Design review of the part shown in the three views and the two pictorial views. Dimensions are in mm from the part's minimum x, y and z. A direction names the side the tool comes from. Give positions to 0.01 mm unless a question says otherwise; leave off trailing zeros. Order: outer loops, then holes, each group sorted by start corner. A loop starts at its lowest first (then second) coordinate and runs counter-clockwise, first axis right, second up. Notation, with made-up numbers: (75.5, 37) - (107.5, 37) arc R30 ccw to (107.5, 64) - close; hole circle Ø10 at (18.5, -25.5). An arc over 180 degrees is marked (long way). Put each result on its own line as item: value.
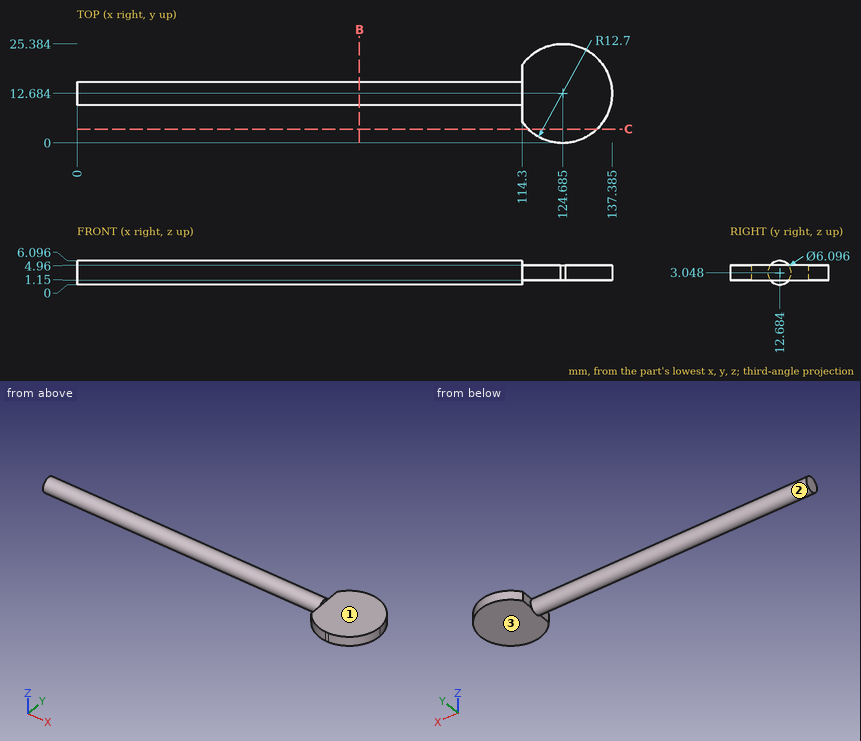
(1) Take a section at C-C, the plane y = 3.5. Write out the cut boundary in (x, z).
The answers:
outline: (115.91, 1.15) - (133.46, 1.15) - (133.46, 4.96) - (115.91, 4.96) - close
(2) Wall thickness on L1, parallel to Z at x = 110.5, y = 13; L2, parallel to Z at x = 119.5, y = 22.75; L3, parallel to Y at x = 45, z = 3.25 (1 decimal): over which ranges is each line inside the solid? List them lowest first.
The answers:
L1: 0.02 to 6.08
L2: 1.15 to 4.96
L3: 9.6 to 15.7
(3) Take a section at B-B, the plane x = 72.5. Write out the cut boundary in (y, z).
The answers:
outline: circle Ø6.1 at (12.68, 3.05)
(4) Clearance check with flat-ended pins moving along their axes: pin 1 Ø11.5 at (x, y) = (128.5, 16) entering from -Z; pin 2 Ø1.1 at (y, z) = (7.5, 3.5) entering from -X; pin 3 Ø1.5 at (x, z) = (35, 5) entering from +Y (1 decimal). State where each tip first meets the part, or that it passes through.
The answers:
pin 1: z = 1.15
pin 2: x = 114.3
pin 3: y = 15.5
(5) For the marked faces 1, 2 and 3, list the 3-axis set-ups (+Z, -Z, +X, -X, +Y, -Y) from which the entire face can be reached by the end or side of a thin tool; tool diameter is ignored.
The answers:
face 1: +Z, +X, +Y, -Y
face 2: -X
face 3: -Z, +X, +Y, -Y
